from build123d import *

# Parameters (mm, degrees)
F1_DEPTH = 14
F2_DEPTH = 18
F3_DEPTH = 4


with BuildPart() as f1:
    # F0 (on Top) → F1 (new body)
    with BuildSketch(Plane.XY):
        Polygon((42.077698, 24.113634), (0.155829, 48.497172), (-41.921869, 24.383538), (-42.077698, -24.113634), (-0.155829, -48.497172), (41.921869, -24.383538), align=None)
        Polygon((-40, 23.094011), (0, 46.188022), (40, 23.094011), (40, -23.094011), (0, -46.188022), (-40, -23.094011), align=None, mode=Mode.SUBTRACT)
    extrude(amount=F1_DEPTH)

    # F0 (on Top) → F2 (join)
    with BuildSketch(Plane.XY):
        Polygon((40, 23.094011), (0, 46.188022), (-40, 23.094011), (-40, -23.094011), (0, -46.188022), (40, -23.094011), align=None)
        Polygon((-12.855593, -8.712208), (-0.855593, -15.640412), (-0.855593, -29.496818), (-12.855593, -36.425021), (-24.855593, -29.496818), (-24.855593, -15.640412), align=None, mode=Mode.SUBTRACT)
        Polygon((13.144407, -8.6083), (25.144407, -15.536503), (25.144407, -29.392909), (13.144407, -36.321113), (1.144407, -29.392909), (1.144407, -15.536503), align=None, mode=Mode.SUBTRACT)
        Polygon((-25.765606, 13.856406), (-13.765606, 6.928203), (-13.765606, -6.928203), (-25.765606, -13.856406), (-37.765606, -6.928203), (-37.765606, 6.928203), align=None, mode=Mode.SUBTRACT)
        Polygon((-12.882803, 36.440731), (-0.882803, 29.512527), (-0.882803, 15.656121), (-12.882803, 8.727918), (-24.882803, 15.656121), (-24.882803, 29.512527), align=None, mode=Mode.SUBTRACT)
        Polygon((0, 13.856406), (12, 6.928203), (12, -6.928203), (0, -13.856406), (-12, -6.928203), (-12, 6.928203), align=None, mode=Mode.SUBTRACT)
        Polygon((13.117197, 36.305403), (25.117197, 29.3772), (25.117197, 15.520794), (13.117197, 8.59259), (1.117197, 15.520794), (1.117197, 29.3772), align=None, mode=Mode.SUBTRACT)
        Polygon((26.234394, 13.856406), (38.234394, 6.928203), (38.234394, -6.928203), (26.234394, -13.856406), (14.234394, -6.928203), (14.234394, 6.928203), align=None, mode=Mode.SUBTRACT)
    extrude(amount=F2_DEPTH)

    # F0 (on Top) → F3 (join)
    with BuildSketch(Plane.XY):
        Polygon((25.117197, 15.520794), (25.117197, 29.3772), (13.117197, 36.305403), (1.117197, 29.3772), (1.117197, 15.520794), (13.117197, 8.59259), align=None)
        Polygon((-0.882803, 15.656121), (-0.882803, 29.512527), (-12.882803, 36.440731), (-24.882803, 29.512527), (-24.882803, 15.656121), (-12.882803, 8.727918), align=None)
        Polygon((-13.765606, -6.928203), (-13.765606, 6.928203), (-25.765606, 13.856406), (-37.765606, 6.928203), (-37.765606, -6.928203), (-25.765606, -13.856406), align=None)
        Polygon((12, -6.928203), (12, 6.928203), (0, 13.856406), (-12, 6.928203), (-12, -6.928203), (0, -13.856406), align=None)
        Polygon((38.234394, -6.928203), (38.234394, 6.928203), (26.234394, 13.856406), (14.234394, 6.928203), (14.234394, -6.928203), (26.234394, -13.856406), align=None)
        Polygon((25.144407, -29.392909), (25.144407, -15.536503), (13.144407, -8.6083), (1.144407, -15.536503), (1.144407, -29.392909), (13.144407, -36.321113), align=None)
        Polygon((-0.855593, -29.496818), (-0.855593, -15.640412), (-12.855593, -8.712208), (-24.855593, -15.640412), (-24.855593, -29.496818), (-12.855593, -36.425021), align=None)
    extrude(amount=F3_DEPTH)


solid = f1.part
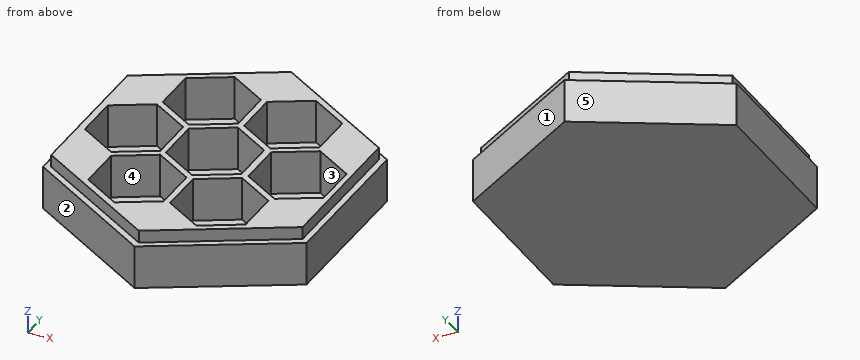
For this review, take the finished solid that the model builds, in its own axes (mm). Face numbers are marked on the shaded views. A direction names the side the tool comes from. Give positions to 0.01 mm unless a question says otherwise; leave off trailing zeros. Loops run counter-clockwise (first coordinate to the right, second up) from the corner with the lowest first, then second, coordinate; pieces in that order, holes last.
Item 1: For line 1 along X through (y, z) = (-4, 14.75); line 2 along X through (y, z) = (-24, 6.25); line 3 along X through (y, z) = (-13, 5.5), list the stretches that pass through material, from the lowest coordinate up.
Item 2: Take a section at D-D, the plane x = 6. State the section outline as (y, z) points, and give its area (3 significant figures).
Item 3: Take a section at C-C, the plane y = -2.5. State the section outline as (x, z) points, and give its area (3 significant figures).
Item 4: Take a section at A-A, the plane z = 16. Give the number of separate pieces and of enclosed holes in the cut face, and give its area (3 significant figures).
Item 5: Tool access review of the marked faces 4 and 5: name each direction out of +Z, -Z, +X, -X, +Y, -Y from which nothing blocks a thin tool from reaching the whole face with its end or side.
Item 6: Take a section at B-B, the plane x = 37. State the section outline as (y, z) points, and give its area (3 significant figures).
Item 7: Insertion check: pin 1 (10 mm diameter, centred on y = 13.5, z = 3, fed in from -X); pin 2 (7 mm diameter, centred on y = 21.5, z = 12.5, fed in from +X); pin 3 (1.2 mm diameter, centred on y = -4.5, z = 16, fed in from +X); pin 4 (10 mm diameter, centred on x = -25, y = 4, fed in from +Z). Each pin has a flat end and moves straight along its axis. Give the tip position at first contact, or say it passes through.
Item 8: Draft analysis for pull direction X (two halves, no side actions). For the marked faces 1, 2 and 3, state which applies: +X half, -X half, draft (parallel to the pull), parting line (faces both ways), or undercut.
Calculated:
1. line 1: x = -40 to -37.77, -13.77 to -12, 12 to 14.23, 38.23 to 40
1. line 2: x = -42.08 to -24.86, -0.86 to 1.14, 25.14 to 41.92
1. line 3: x = -42.04 to -27.25, -24.28 to -20.28, -5.43 to -1.48, 1.48 to 5.54, 20.75 to 24.75, 27.72 to 41.96
2. outline: (-44.97, 0) - (45.1, 0) - (45.1, 14) - (42.72, 14) - (42.72, 18) - (32.2, 18) - (32.2, 4) - (12.7, 4) - (12.7, 18) - (10.39, 18) - (10.39, 4) - (-10.39, 4) - (-10.39, 18) - (-12.73, 18) - (-12.73, 4) - (-32.2, 4) - (-32.2, 18) - (-42.72, 18) - (-42.72, 14) - (-44.97, 14) - close
2. area: 766 mm2
3. outline: (-42.01, 0) - (41.99, 0) - (41.99, 14) - (40, 14) - (40, 18) - (38.23, 18) - (38.23, 4) - (14.23, 4) - (14.23, 18) - (12, 18) - (12, 4) - (-12, 4) - (-12, 18) - (-13.77, 18) - (-13.77, 4) - (-37.77, 4) - (-37.77, 18) - (-40, 18) - (-40, 14) - (-42.01, 14) - close
3. area: 488 mm2
4. separate pieces: 1
4. enclosed holes: 7
4. area: 2,050 mm2
5. face 4: +Z
5. face 5: +Z, -Z, -X, +Y
6. outline: (-27.2, 0) - (27.07, 0) - (27.07, 14) - (24.83, 14) - (24.83, 18) - (7.64, 18) - (7.64, 4) - (-7.64, 4) - (-7.64, 18) - (-24.83, 18) - (-24.83, 14) - (-27.2, 14) - close
6. area: 744 mm2
7. pin 1: stops at x = -41.97
7. pin 2: stops at x = 42.08
7. pin 3: stops at x = 40
7. pin 4: stops at z = 4
8. face 1: +X half
8. face 2: -X half
8. face 3: undercut
